```python
from build123d import *

# Parameters (mm, degrees)
CROQUIS1_R              = 10.668
SALIENTE_EXTRUIR1_DEPTH = 5
CORTAR_EXTRUIR1_REACH   = 55.921
CROQUIS2_R              = 2.25
SALIENTE_EXTRUIR2_DEPTH = 2.5
CROQUIS7_W              = 2
CROQUIS7_H              = 8
CORTAR_EXTRUIR5_DEPTH   = 55.612046519
SALIENTE_EXTRUIR3_DEPTH = 10
CORTAR_EXTRUIR6_REACH   = 65.994
CROQUIS9_R              = 2.25


with BuildPart() as part:
    # Croquis1 → Saliente-Extruir1 (new, symmetric)
    with BuildSketch(Plane(origin=(0, 0, 0), x_dir=(1, 0, 0), z_dir=(0, 1, 0))):
        with BuildLine():
            Line((30, 0), (-30, 0))
            Line((-30, 0), (-30, -10))
            Line((-30, -10), (-5, -10))
            Line((-5, -10), (-5, -16.362711963))
            ThreePointArc((-5, -16.362711963), (0, -44.525), (5, -16.362711963))
            Line((5, -16.362711963), (5, -10))
            Line((5, -10), (30, -10))
            Line((30, -10), (30, 0))
        make_face()
        with Locations(Location((0, -30, 0), (0, 0, 270))):
            Circle(CROQUIS1_R, mode=Mode.SUBTRACT)
    extrude(amount=SALIENTE_EXTRUIR1_DEPTH, both=True)

    # Croquis2 → Cortar-Extruir1 (cut, up to next)
    with BuildSketch(Plane(origin=(0, 0, 0), x_dir=(-1, 0, 0), z_dir=(0, 0, -1)), mode=Mode.PRIVATE) as cortar_extruir1_sk1:
        with Locations((25, 0)):
            Circle(CROQUIS2_R)
    cortar_extruir1_tool1 = extrude(cortar_extruir1_sk1.sketch, amount=-CORTAR_EXTRUIR1_REACH, mode=Mode.PRIVATE) & part.part
    # Croquis2 → Cortar-Extruir1 (cut, up to next)
    with BuildSketch(Plane(origin=(0, 0, 0), x_dir=(-1, 0, 0), z_dir=(0, 0, -1)), mode=Mode.PRIVATE) as cortar_extruir1_sk2:
        with Locations((-25, 0)):
            Circle(CROQUIS2_R)
    cortar_extruir1_tool2 = extrude(cortar_extruir1_sk2.sketch, amount=-CORTAR_EXTRUIR1_REACH, mode=Mode.PRIVATE) & part.part
    add(cortar_extruir1_tool1.solids().sort_by_distance((-25, 0, 0))[0], mode=Mode.SUBTRACT)
    add(cortar_extruir1_tool2.solids().sort_by_distance((25, 0, 0))[0], mode=Mode.SUBTRACT)

    # Croquis3 → Saliente-Extruir2 (add, symmetric)
    with BuildSketch(Plane(origin=(0, 0, 0), x_dir=(1, 0, 0), z_dir=(0, 1, 0))):
        with BuildLine():
            ThreePointArc((-5, -16.362711963), (-12.838793561, -23.207282952), (-14.0873706, -33.53858935))
            Line((-14.0873706, -33.53858935), (-20, -10))
            Line((-20, -10), (-5, -10))
            Line((-5, -10), (-5, -16.362711963))
        make_face()
        with BuildLine():
            Line((5, -10), (5, -16.362711963))
            ThreePointArc((5, -16.362711963), (12.838793561, -23.207282952), (14.0873706, -33.53858935))
            Line((14.0873706, -33.53858935), (20, -10))
            Line((20, -10), (5, -10))
        make_face()
    extrude(amount=SALIENTE_EXTRUIR2_DEPTH, both=True)

    # Croquis7 → Cortar-Extruir5 (cut, through all)
    with BuildSketch(Plane(origin=(0, 5, 0), x_dir=(1, 0, 0), z_dir=(0, 1, 0))):
        with Locations((0, -42.5965)):
            Rectangle(CROQUIS7_W, CROQUIS7_H)
    extrude(amount=-CORTAR_EXTRUIR5_DEPTH, mode=Mode.SUBTRACT)

    # Croquis8 → Saliente-Extruir3 (add)
    with BuildSketch(Plane(origin=(0, 5, 0), x_dir=(1, 0, 0), z_dir=(0, 1, 0))):
        with BuildLine():
            Line((-1, -44.490535704), (-1, -50.490535704))
            Line((-1, -50.490535704), (-9, -50.490535704))
            Line((-9, -50.490535704), (-9, -41.400685286))
            ThreePointArc((-9, -41.400685286), (-5.233239332, -43.549495603), (-1, -44.490535704))
        make_face()
        with BuildLine():
            Line((9, -50.490535704), (9, -41.400685286))
            ThreePointArc((9, -41.400685286), (5.233239332, -43.549495603), (1, -44.490535704))
            Line((1, -44.490535704), (1, -50.490535704))
            Line((1, -50.490535704), (9, -50.490535704))
        make_face()
    extrude(amount=-SALIENTE_EXTRUIR3_DEPTH)

    # Cortar-Extruir6: up to this face of the body (flat: up to its plane)
    cortar_extruir6_end = Plane(part.part.faces().sort_by_distance((-9, 0, 45.945610495))[0])
    # Croquis9 → Cortar-Extruir6 (cut, up to the picked face)
    with BuildSketch(Plane(origin=(9, 0, 0), x_dir=(0, 0, -1), z_dir=(1, 0, 0)), mode=Mode.PRIVATE) as cortar_extruir6_sk1:
        with Locations((-45.945610495, 0)):
            Circle(CROQUIS9_R)
    cortar_extruir6_tool1 = split(extrude(cortar_extruir6_sk1.sketch, amount=-CORTAR_EXTRUIR6_REACH, mode=Mode.PRIVATE), bisect_by=cortar_extruir6_end, keep=Keep.BOTH, mode=Mode.PRIVATE)
    add(cortar_extruir6_tool1.solids().sort_by(Axis((9, 0, 45.94561), (-1, 0, 0)))[0], mode=Mode.SUBTRACT)


solid = part.part
```
Verification items for the finished model (mm, model axes). A direction names the side the tool comes from. Coordinates: 2 decimals unless noted, no trailing zeros. Loops run counter-clockwise (first coordinate to the right, second up) from the corner with the lowest first, then second, coordinate; pieces in that order, holes last. Notation, with made-up numbers: (4.25, -31.75) -> (11.25, -31.75) arc R27 ccw to (11.25, 2.25) -> close; hole circle Ø9 at (81, -16). An arc over 180 degrees is marked (long way). Answer in a Markdown table with one row per item.
1) Section check D-D (z = 8). Record the cut outline in (x, y).
The answers:
| item | result |
|---|---|
| outline | (-30, -5) -> (30, -5) -> (30, 5) -> (-30, 5) -> close; hole circle Ø4.5 at (-25, 0); hole circle Ø4.5 at (25, 0) |
2) Access from +Z, -Z, +X, -X, +Y, -Y to the whole of each face (thin tool, end or side, straight path). Record for faces 1 (the face through (-12, 2.5, 16)), 2 (the face through (-1, 0, 43)), 3 (the face through (13.75, 0.07, 34.68)), 4 (the face through (12, -2.5, 16)), 5 (the face through (-5, -4, 13)).
The answers:
| item | result |
|---|---|
| face 1 | -X, +Y |
| face 2 | +Z, +Y, -Y |
| face 3 | +X |
| face 4 | +X, -Y |
| face 5 | -X, -Y |
3) Section check C-C (x = -6). Record the cut outline in (y, z).
The answers:
| item | result |
|---|---|
| outline | (-5, 0) -> (5, 0) -> (5, 10) -> (2.5, 10) -> (2.5, 16.77) -> (5, 16.77) -> (5, 21.18) -> (-5, 21.18) -> (-5, 16.77) -> (-2.5, 16.77) -> (-2.5, 10) -> (-5, 10) -> close; (-5, 38.82) -> (5, 38.82) -> (5, 50.49) -> (-5, 50.49) -> close; hole circle Ø4.5 at (0, 45.95) |
4) Scan lines: line 1 along X through (y, z) = (2, 42.5); line 2 along X through (y, z) = (4.25, 29.5); line 3 along Y through (x, z) = (25, 6). Record each from-to range of solid material in increasing order. Write a range as from..to.
The answers:
| item | result |
|---|---|
| line 1 | x = -9..-1, 1..9 |
| line 2 | x = -14.52..-10.66, 10.66..14.52 |
| line 3 | y = -5..-2.25, 2.25..5 |
5) Draft check along Z on faces 6 (the face through (22.854, 0.676, 4.93)), 7 (the face through (5, -4, 13)), 8 (the face through (12, 2.5, 16)), 9 (the face through (5, 0, 50.491)). Enter one of: released by +Z, released by -Z, zero draft, split by the parting line, or undercut.
The answers:
| item | result |
|---|---|
| face 6 | zero draft |
| face 7 | undercut |
| face 8 | undercut |
| face 9 | released by +Z |
6) Section check A-A (x = -25). Record the cut outline in (y, z), and give its area (3 significant figures).
The answers:
| item | result |
|---|---|
| outline | (-5, 0) -> (-2.25, 0) -> (-2.25, 10) -> (-5, 10) -> close; (2.25, 0) -> (5, 0) -> (5, 10) -> (2.25, 10) -> close |
| area | 55.0 mm2 |
7) Section check B-B (y = 0). Give the number of separate pieces and of enclosed holes in the cut face, and give its area (3 significant figures).
The answers:
| item | result |
|---|---|
| separate pieces | 5 |
| enclosed holes | 0 |
| area | 1,220 mm2 |
8) Depth check by flat-ended pin: P1, Ø4, axis at x = -15.5, y = -3, coming from the -Z side; P2, Ø5, axis at x = 25, y = 0, coming from the +Z side; P3, Ø19, axis at x = 0, z = 30, coming from the +Y side; P4, Ø0.8, axis at y = 3.5, z = 14, coming from the -X side. Enter the tip coordinate at first touch or a pass-through.
The answers:
| item | result |
|---|---|
| P1 | stops at z = 0 |
| P2 | stops at z = 10 |
| P3 | passes through |
| P4 | stops at x = -5 |
